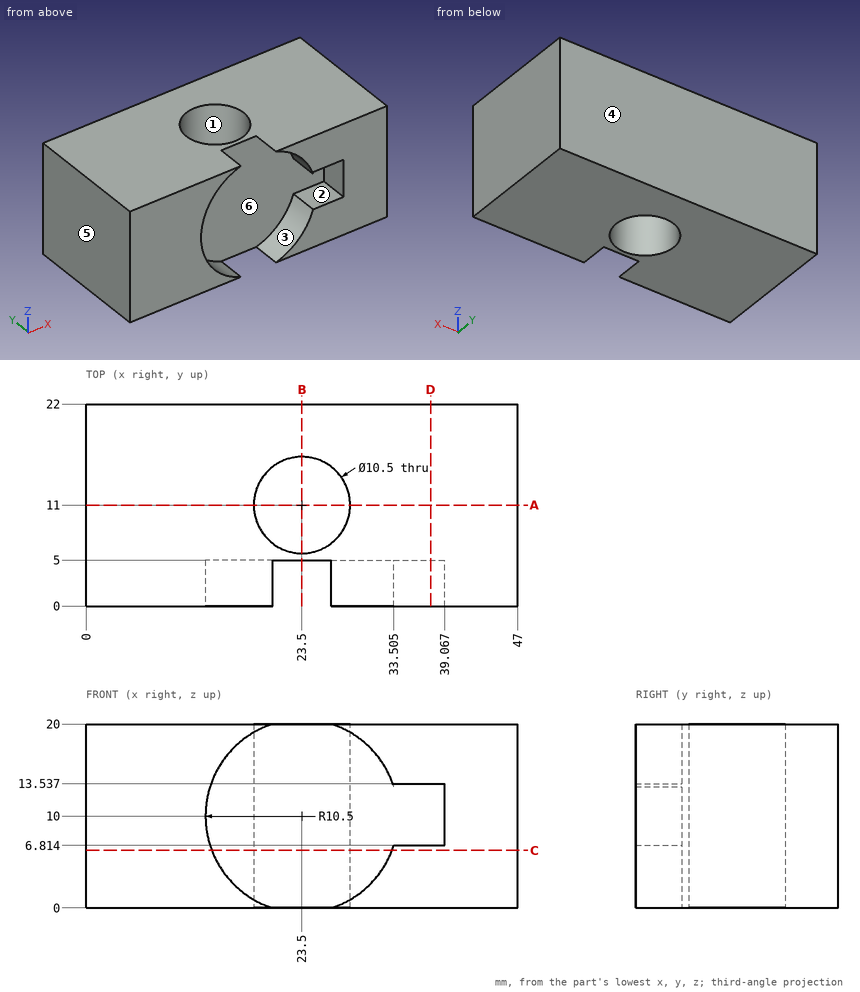
Geometry: see drawing. Coordinates: mm, zero at the bounding-box minimum. A direction names the side the tool comes from. Coordinates: 2 decimals unless noted, no trailing zeros. Loops run counter-clockwise (first coordinate to the right, second up) from the corner with the lowest first, then second, coordinate; pieces in that order, holes last. Notation, with made-up numbers: (9, 85) - (27, 85) arc R23 ccw to (27, 113) - close; hole circle Ø4 at (14.25, 58). An arc over 180 degrees is marked (long way). Answer as CSV lines item,"result".
1. Section D-D (x = 37.5). Return loops of the section in (y, z).
Established:
outline,"(0, 0) - (22, 0) - (22, 20) - (0, 20) - (0, 13.54) - (5, 13.54) - (5, 6.81) - (0, 6.81) - close"
2. Mould query, pull axis X, two halves, no side actions, for the marked faces 3, 4, 5 and 6. Classes: released by +X, released by -X, zero draft, split by the parting line, or undercut.
Established:
face 3,"undercut"
face 4,"zero draft"
face 5,"released by -X"
face 6,"undercut"
3. Reachability of the marked faces 1 and 2 from +Z, -Z, +X, -X, +Y, -Y: full face, straight path, thin tool, end or side. Return the list, or none.
Established:
face 1,"+Z, -Z"
face 2,"-Y"
4. Section C-C (z = 6.25). Return loops of the section in (x, y).
Established:
outline,"(0, 0) - (13.69, 0) - (13.69, 5) - (33.31, 5) - (33.31, 0) - (47, 0) - (47, 22) - (0, 22) - close; hole circle Ø10.5 at (23.5, 11)"
5. Section B-B (x = 23.5). Return loops of the section in (y, z), then the cut area to 3 significant figures.
Established:
outline,"(5, 0) - (5.75, 0) - (5.75, 20) - (5, 20) - close; (16.25, 0) - (22, 0) - (22, 20) - (16.25, 20) - close"
area,"130 mm2"
6. Ray query, line 1 (Y direction, x = 23.5, z = 6.5); line 2 (Z direction, x = 34, y = 3); line 3 (X direction, y = 10.75, z = 16.5) (1 decimal). Return the intervals inside material, ascending.
Established:
line 1,"y = 5 to 5.75, 16.25 to 22"
line 2,"z = 0 to 6.81, 13.54 to 20"
line 3,"x = 0 to 18.3, 28.7 to 47"
7. Section A-A (y = 11). Return loops of the section in (x, z).
Established:
outline,"(0, 0) - (18.25, 0) - (18.25, 20) - (0, 20) - close; (28.75, 0) - (47, 0) - (47, 20) - (28.75, 20) - close"
